Check sheet for the modelled part. Datum: model origin and axes. Units: mm. A direction names the side the tool comes from. Give positions to 0.01 mm unless a question says otherwise; leave off trailing zeros. Order: outer loops, then holes, each group sorted by start corner. A loop starts at its lowest first (then second) coordinate and runs counter-clockwise, first axis right, second up.
Item 1: Gauge pin test, flat ends, axial feed: P1, Ø1, axis at y = 5, z = -1, coming from the -X side; P2, Ø1.5, axis at y = 4.5, z = 5.5, coming from the +X side. Record the tip position at first contact, or that the pin passes through.
Item 2: Material ranges on line 1 along Z through (x, y) = (2.25, 5); line 2 along X through (y, z) = (5.5, -3.5); line 3 along Z through (x, y) = (9.25, 6.75), recorded low to high.
Item 3: Sectioned sample at A-A on x = 3.5. Record the boundary of the cut face in (y, z) (3 decimals), and give its area (3 significant figures).
Item 4: Access from +Z, -Z, +X, -X, +Y, -Y to the whole of each face (thin tool, end or side, straight path). Record for faces 4 (the flat face through (0, 5, -11.758)), 5 (the flat face through (5.742, 4.696, -3.253)).
Item 5: Sectioned sample at B-B on y = 1.75. Record the boundary of the cut face in (x, z).
Item 6: Release check for a two-part mould opening along Y. For faces 1 (the flat face through (-6.2, 0, -2.8)), 2 (the flat face through (10.23, 4.7, -5.8)), 3 (the cylindrical face through (9.34, 7.22, 5.77)) record: released by +Y, released by -Y, zero draft, split by the parting line, or undercut.
Item 7: Sectioned sample at D-D on y = 5.5. Record the boundary of the cut face in (x, z).
Item 8: Sectioned sample at C-C on z = 1.25. Record the boundary of the cut face in (x, y) (3 decimals), and give its area (3 significant figures).
from build123d import *

# Parameters (mm, degrees)
BOSS_EXTRUDE1_DEPTH = 9.525
SKETCH2_R           = 2.48046875
CUT_EXTRUDE1_DEPTH  = 1.5875
SKETCH3_R           = 1.5875
CUT_EXTRUDE2_DEPTH  = 6.35
SKETCH4_R           = 2.45760875
CUT_EXTRUDE3_DEPTH  = 1.5875
CUT_EXTRUDE4_START  = -6.35
SKETCH5_R           = 1.5875
CUT_EXTRUDE4_DEPTH  = 6.35


with BuildPart() as part:
    # Sketch1 → Boss-Extrude1 (new body)
    with BuildSketch(Plane(origin=(0, 0, 0), x_dir=(1, 0, 0), z_dir=(0, 1, 0))):
        Polygon((13.57753309, 0), (6.788766545, 11.758488577), (-6.788766545, 11.758488577), (-13.57753309, 0), (-6.788766545, -11.758488577), (6.788766545, -11.758488577), align=None)
        Polygon((7.62, 0), (3.81, 6.599113577), (-3.81, 6.599113577), (-7.62, 0), (-3.81, -6.599113577), (3.81, -6.599113577), align=None, mode=Mode.SUBTRACT)
    extrude(amount=BOSS_EXTRUDE1_DEPTH)

    # Sketch2 → Cut-Extrude1 (cut)
    with BuildSketch(Plane(origin=(10.183149818, 0, 5.879244288), x_dir=(0.4999999999999997, 0, -0.8660254037844389), z_dir=(0.8660254037844389, 0, 0.4999999999999997))):
        with Locations((0, 4.7625)):
            Circle(SKETCH2_R)
    extrude(amount=-CUT_EXTRUDE1_DEPTH, mode=Mode.SUBTRACT)

    # Sketch3 → Cut-Extrude2 (cut)
    with BuildSketch(Plane(origin=(8.808334489, 0, 5.085494288), x_dir=(0.49999999999999983, 0, -0.8660254037844388), z_dir=(0.8660254037844387, 0, 0.4999999999999998))):
        with Locations((0, 4.7625)):
            Circle(SKETCH3_R)
    extrude(amount=-CUT_EXTRUDE2_DEPTH, mode=Mode.SUBTRACT)

    # Sketch4 → Cut-Extrude3 (cut)
    with BuildSketch(Plane(origin=(-10.183149818, 0, -5.879244288), x_dir=(-0.4999999999999997, 0, 0.8660254037844389), z_dir=(-0.8660254037844389, 0, -0.4999999999999997))):
        with Locations((0, 4.7625)):
            Circle(SKETCH4_R)
    extrude(amount=-CUT_EXTRUDE3_DEPTH, mode=Mode.SUBTRACT)

    # Sketch5 → Cut-Extrude4 (cut)
    with BuildSketch(Plane(origin=(-8.808334489, 0, -5.085494288), x_dir=(-0.49999999999999983, 0, 0.8660254037844388), z_dir=(-0.8660254037844387, 0, -0.4999999999999998)).offset(CUT_EXTRUDE4_START)):
        with Locations(Location((0, 4.7625, 0), (0, 0, 180))):
            Circle(SKETCH5_R)
    extrude(amount=CUT_EXTRUDE4_DEPTH, mode=Mode.SUBTRACT)


solid = part.part
Report:
1. P1: stops at x = -13.29
1. P2: stops at x = 7.75
2. line 1: z = -11.76 to -6.6, 6.6 to 11.76
2. line 2: x = -11.56 to -10.75, -9.72 to -8.87, 5.6 to 11.56
2. line 3: z = -7.5 to 4.32, 7.05 to 7.5
3. outline: (0, -11.758) - (9.525, -11.758) - (9.525, -6.599) - (0, -6.599) - close; (0, 6.599) - (9.525, 6.599) - (9.525, 11.758) - (0, 11.758) - close
3. area: 98.3 mm2
4. face 4: -Z, +X, -X, +Y, -Y
4. face 5: +Y, -Y
5. outline: (-13.58, 0) - (-6.79, -11.76) - (6.79, -11.76) - (13.58, 0) - (6.79, 11.76) - (-6.79, 11.76) - close; hole (-7.62, 0) - (-3.81, -6.6) - (3.81, -6.6) - (7.62, 0) - (3.81, 6.6) - (-3.81, 6.6) - close
6. face 1: released by -Y
6. face 2: zero draft
6. face 3: undercut
7. outline: (-13.58, 0) - (-11.36, -3.85) - (-9.98, -3.06) - (-9.51, -3.87) - (-6.42, -2.08) - (-7.62, 0) - (-3.81, 6.6) - (3.81, 6.6) - (5.01, 4.52) - (8.11, 6.3) - (7.62, 7.14) - (9, 7.93) - (6.79, 11.76) - (-6.79, 11.76) - close; (-9.01, -7.91) - (-6.79, -11.76) - (6.79, -11.76) - (13.58, 0) - (11.37, 3.83) - (9.99, 3.03) - (9.51, 3.87) - (6.42, 2.08) - (7.62, 0) - (3.81, -6.6) - (-3.81, -6.6) - (-5.01, -4.52) - (-8.11, -6.3) - (-7.64, -7.12) - close
8. outline: (-12.856, 0) - (-6.898, 0) - (-6.898, 9.525) - (-12.856, 9.525) - close; (6.898, 0) - (12.856, 0) - (12.856, 9.525) - (6.898, 9.525) - close
8. area: 113 mm2
